```python
from build123d import *

# Parameters (mm, degrees)
SKETCH005_W             = 33.5
SKETCH005_H             = 18
PAD006_DEPTH            = 1.5
BOX013_W                = 5.5
BOX013_H                = 8
BOX013_DEPTH            = 2.5
BOX014_W                = 7.5
BOX014_H                = 7.5
BOX014_DEPTH            = 1
BODY008_PLACEMENT_ANGLE = 180


with BuildPart() as part:
    # Sketch005 → Pad006 (new body)
    with BuildSketch(Plane.XZ):
        with Locations((16.75, 9)):
            Rectangle(SKETCH005_W, SKETCH005_H)
    extrude(amount=PAD006_DEPTH)

    # Box013 → Box013 (join)
    with BuildSketch(Plane(origin=(-1, 2.5, 5), x_dir=(1, 0, 0), z_dir=(0, -1, 0))):
        with Locations((2.75, 4)):
            Rectangle(BOX013_W, BOX013_H)
    extrude(amount=BOX013_DEPTH)

    # Box014 → Box014 (join)
    with BuildSketch(Plane(origin=(19, 1, 3.7), x_dir=(0.707107, 0, 0.707107), z_dir=(0, -1, 0))):
        with Locations((3.75, 3.75)):
            Rectangle(BOX014_W, BOX014_H)
    extrude(amount=BOX014_DEPTH)


with BuildPart() as part_1:
    # Body008 placement: moved
    add(part.part.moved(Location((0, -6, 69))).rotate(Axis((0, -6, 69), (1, 0, 0)), BODY008_PLACEMENT_ANGLE))


solid = part_1.part
```
Build history of the part. All positions in model axes, mm. A direction names the side the tool comes from. Round coordinates to 2 decimals unless told otherwise and drop trailing zeros. Order: outer loops, then holes, each group sorted by start corner. A loop starts at its lowest first (then second) coordinate and runs counter-clockwise, first axis right, second up. Notation, with made-up numbers: (-18, -25) -> (19, -25) arc R32 cw to (19, 10) -> close; hole circle Ø11 at (82, 54.5). An arc over 180 degrees is marked (long way). Answer in a Markdown table with one row per item.
1) Pin check, flat tips, straight feed: P1, Ø1.5, axis at y = -7.5, z = 56.5, coming from the +X side; P2, Ø1.7, axis at y = -5.5, z = 62.5, coming from the -X side; P3, Ø1.3, axis at y = -7.5, z = 59, coming from the +X side; P4, Ø3, axis at x = 20.5, z = 59, coming from the -Y side. Stop position of each tip, or through.
Values:
| item | result |
|---|---|
| P1 | x = 21.37 |
| P2 | x = -1 |
| P3 | x = 23.72 |
| P4 | y = -7 |
2) Which spindle directions (+Z, -Z, +X, -X, +Y, -Y) get a long thin tool onto all of the face, cutting with end or side? Do faces 5 (the flat face through (19, -7, 60)), 6 (the flat face through (-0.5, -6, 59.9)), 7 (the flat face through (21.689, -6.507, 57.382)). Say none if no direction does.
Values:
| item | result |
|---|---|
| face 5 | +Z, -Z, +X, -Y |
| face 6 | +Z, -Z, -X, +Y |
| face 7 | -Z, +X, -Y |
3) Band-saw the part on D-D on z = 58. Give the cut face in (x, y), and give its area (3 significant figures).
Values:
| item | result |
|---|---|
| outline | (-1, -8.5) -> (4.5, -8.5) -> (4.5, -6) -> (15.69, -6) -> (15.69, -7) -> (22.31, -7) -> (22.31, -6) -> (33.5, -6) -> (33.5, -4.5) -> (0, -4.5) -> (0, -6) -> (-1, -6) -> close |
| area | 70.6 mm2 |
4) Band-saw the part on C-C on x = 22.5. Give the cut face in (y, z).
Values:
| item | result |
|---|---|
| outline | (-7, 58.19) -> (-6, 58.19) -> (-6, 51) -> (-4.5, 51) -> (-4.5, 69) -> (-6, 69) -> (-6, 61.8) -> (-7, 61.8) -> close |
5) Band-saw the part on A-A on z = 61.75. Give the cut face in (x, y).
Values:
| item | result |
|---|---|
| outline | (-1, -8.5) -> (4.5, -8.5) -> (4.5, -6) -> (15.45, -6) -> (15.45, -7) -> (22.55, -7) -> (22.55, -6) -> (33.5, -6) -> (33.5, -4.5) -> (0, -4.5) -> (0, -6) -> (-1, -6) -> close |
6) Mould opens along X. For faces 1 (the flat face through (21.6, -6.5, 62.7)), 2 (the flat face through (2, -8.5, 60)), 3 (the flat face through (17, -6, 56)), 4 (the flat face through (0, -5, 60)) say: released by +X, released by -X, zero draft, split by the parting line, or undercut.
Values:
| item | result |
|---|---|
| face 1 | released by +X |
| face 2 | zero draft |
| face 3 | undercut |
| face 4 | released by -X |
7) Band-saw the part on B-B on y = -4.9. Give the cut face in (x, z), and give its area (3 significant figures).
Values:
| item | result |
|---|---|
| outline | (0, 51) -> (33.5, 51) -> (33.5, 69) -> (0, 69) -> close |
| area | 603 mm2 |
8) Wall check: L1, parallel to Y at x = 17.5, z = 61; L2, parallel to Y at x = 9.5, z = 64.25; L3, parallel to X at y = -6.75, z = 63. Give the ranges that are in metal, low to high.
Values:
| item | result |
|---|---|
| L1 | -7 to -4.5 |
| L2 | -6 to -4.5 |
| L3 | -1 to 4.5, 16.7 to 21.3 |
